Here's how the part is built. I have some questions about the finished solid (model axes, mm). A direction names the side the tool comes from. Coordinates: 2 decimals unless noted, no trailing zeros. Order: outer loops, then holes, each group sorted by start corner. A loop starts at its lowest first (then second) coordinate and runs counter-clockwise, first axis right, second up. Notation, with made-up numbers: (86, -33) - (144, -33) arc R32 cw to (144, 6) - close; hole circle Ø10 at (80.25, 13.5). An arc over 180 degrees is marked (long way). Answer in a Markdown table with one row per item. Add a question column.
Item 1: I want a section at C-C (x = -41). Please give me the cut outline in (y, z).
Item 2: I want a section at B-B (z = 1.2). Please give me the cut outline in (x, y).
Item 3: Thinking about a two-plate mould opening in X: for faces 3 (the cylindrical face through (-3.01, 2.85, 1.48)), 4 (the cylindrical face through (-69.4, 4.57, 1.48)), 5 (the cylindrical face through (-76.99, 57.15, 1.48)), which applies, +X half, -X half, draft (parallel to the pull), parting line (faces both ways), or undercut?
Item 4: On a 3-axis mill with a long thin cutter (end or side, diameter ignored), from which of +Z, -Z, +X, -X, +Y, -Y can I reach the whole of each face in a straight line? I mean faces 1 (the flat face through (-64, 24, 1)), 2 (the flat face through (-41, 17, 3)). Say none if no direction works.
Item 5: Will this pin go through, and if not, where does the flat tip stop? pin 1 Ø10 at (x, y) = (-32.5, 43) entering from -Z.
Item 6: If I drill on line 1 along X through (y, z) = (13, 2.35); line 2 along X through (y, z) = (37.5, 1.2); line 3 along X through (y, z) = (8.5, 1.6), over which ranges is the centre line in solid material (lowest first)? Write a range as from..to.
Item 7: I want a section at D-D (y = 38.5). Please give me the cut outline in (x, z), plus the area to 3 significant figures.
Item 8: I want a section at A-A (y = 23.5). Please give me the cut outline in (x, z).
```python
from build123d import *

# Parameters (mm, degrees)
F1_DEPTH = 3


with BuildPart() as f1:
    # F0 (on Top) → F1 (new body)
    with BuildSketch(Plane.XY):
        with BuildLine():
            Line((-67.040354, 0), (-10, 0))
            ThreePointArc((-10, 0), (-2.928932, 2.928932), (0, 10))
            Line((0, 10), (0, 30))
            Line((0, 30), (0, 50))
            ThreePointArc((0, 50), (-2.928932, 57.071068), (-10, 60))
            Line((-10, 60), (-40, 60))
            Line((-40, 60), (-70, 60))
            ThreePointArc((-70, 60), (-77.071068, 57.071068), (-80, 50))
            Line((-80, 50), (-80, 36.222443))
            Line((-80, 36.222443), (-80, 10))
            ThreePointArc((-80, 10), (-77.071068, 2.928932), (-70, 0))
            Line((-70, 0), (-67.040354, 0))
        make_face()
        with BuildLine():
            Line((-66, 4), (-67.040354, 4))
            Line((-67.040354, 4), (-68, 4))
            ThreePointArc((-68, 4), (-69.414214, 4.585786), (-70, 6))
            Line((-70, 6), (-70, 42.1))
            ThreePointArc((-70, 42.1), (-69.414214, 43.514214), (-68, 44.1))
            Line((-68, 44.1), (-66, 44.1))
            ThreePointArc((-66, 44.1), (-64.585786, 43.514214), (-64, 42.1))
            Line((-64, 42.1), (-64, 6))
            ThreePointArc((-64, 6), (-64.585786, 4.585786), (-66, 4))
        make_face(mode=Mode.SUBTRACT)
        with BuildLine():
            Line((-8.297237, 42.15616), (-8.297237, 30))
            Line((-8.297237, 30), (-8.297237, 6.05616))
            ThreePointArc((-8.297237, 6.05616), (-8.883023, 4.641946), (-10.297237, 4.05616))
            Line((-10.297237, 4.05616), (-12.297237, 4.05616))
            ThreePointArc((-12.297237, 4.05616), (-13.71145, 4.641946), (-14.297237, 6.05616))
            Line((-14.297237, 6.05616), (-14.297237, 42.15616))
            ThreePointArc((-14.297237, 42.15616), (-13.71145, 43.570373), (-12.297237, 44.15616))
            Line((-12.297237, 44.15616), (-10.297237, 44.15616))
            ThreePointArc((-10.297237, 44.15616), (-8.883023, 43.570373), (-8.297237, 42.15616))
        make_face(mode=Mode.SUBTRACT)
        with BuildLine():
            ThreePointArc((-22.499999, 37.5), (-52.374367, 25.125631), (-40, 55))
            ThreePointArc((-40, 55), (-27.625631, 49.874369), (-22.499999, 37.5))
        make_face(mode=Mode.SUBTRACT)
    extrude(amount=F1_DEPTH)


solid = f1.part
```
Values follow:
| question | item | result |
|---|---|---|
| 1 | outline | (0, 0) - (20.03, 0) - (20.03, 3) - (0, 3) - close; (54.97, 0) - (60, 0) - (60, 3) - (54.97, 3) - close |
| 2 | outline | (-80, 10) arc R10 ccw to (-70, 0) - (-10, 0) arc R10 ccw to (0, 10) - (0, 50) arc R10 ccw to (-10, 60) - (-70, 60) arc R10 ccw to (-80, 50) - close; hole (-70, 6) arc R2 ccw to (-68, 4) - (-66, 4) arc R2 ccw to (-64, 6) - (-64, 42.1) arc R2 ccw to (-66, 44.1) - (-68, 44.1) arc R2 ccw to (-70, 42.1) - close; hole circle Ø35 at (-40, 37.5); hole (-14.3, 6.06) arc R2 ccw to (-12.3, 4.06) - (-10.3, 4.06) arc R2 ccw to (-8.3, 6.06) - (-8.3, 42.16) arc R2 ccw to (-10.3, 44.16) - (-12.3, 44.16) arc R2 ccw to (-14.3, 42.16) - close |
| 3 | face 3 | +X half |
| 3 | face 4 | undercut |
| 3 | face 5 | -X half |
| 4 | face 1 | +Z, -Z |
| 4 | face 2 | +Z, +X, -X, +Y, -Y |
| 5 | pin 1 | passes through |
| 6 | line 1 | x = -80..-70, -64..-14.3, -8.3..0 |
| 6 | line 2 | x = -80..-70, -64..-57.5, -22.5..-14.3, -8.3..0 |
| 6 | line 3 | x = -79.89..-70, -64..-14.3, -8.3..-0.11 |
| 7 | outline | (-80, 0) - (-70, 0) - (-70, 3) - (-80, 3) - close; (-64, 0) - (-57.47, 0) - (-57.47, 3) - (-64, 3) - close; (-22.53, 0) - (-14.3, 0) - (-14.3, 3) - (-22.53, 3) - close; (-8.3, 0) - (0, 0) - (0, 3) - (-8.3, 3) - close |
| 7 | area | 99.2 mm^2 |
| 8 | outline | (-80, 0) - (-70, 0) - (-70, 3) - (-80, 3) - close; (-64, 0) - (-50.5, 0) - (-50.5, 3) - (-64, 3) - close; (-29.5, 0) - (-14.3, 0) - (-14.3, 3) - (-29.5, 3) - close; (-8.3, 0) - (0, 0) - (0, 3) - (-8.3, 3) - close |
